from build123d import *

# Parameters (mm, degrees)
SKETCH1_R           = 9
BOSS_EXTRUDE1_DEPTH = 1.75
SKETCH2_R           = 1.67
SKETCH2_W           = 4.7
SKETCH2_H           = 4.7
CUT_EXTRUDE1_DEPTH  = 2.75


with BuildPart() as part:
    # Sketch1 → Boss-Extrude1 (new body)
    with BuildSketch(Plane.XY):
        Circle(SKETCH1_R)
    extrude(amount=BOSS_EXTRUDE1_DEPTH)

    # Sketch2 → Cut-Extrude1 (cut, through all)
    with BuildSketch(Plane.XY.offset(1.75)):
        with Locations((0, 5.25)):
            Circle(SKETCH2_R)
        Rectangle(SKETCH2_W, SKETCH2_H)
    extrude(amount=-CUT_EXTRUDE1_DEPTH, mode=Mode.SUBTRACT)


solid = part.part
The listing builds one solid part. Answer for the finished solid, in the listing's coordinates (mm). A direction names the side the tool comes from. Give positions to 0.01 mm unless a question says otherwise; leave off trailing zeros. Loops run counter-clockwise (first coordinate to the right, second up) from the corner with the lowest first, then second, coordinate; pieces in that order, holes last.
Item 1: A cutting plane is placed at A-A (x = 0). Give the vertices of the cut face in (y, z), then the cut area to 3 significant figures.
Derived:
outline: (-9, 0) - (-2.35, 0) - (-2.35, 1.75) - (-9, 1.75) - close; (2.35, 0) - (3.58, 0) - (3.58, 1.75) - (2.35, 1.75) - close; (6.92, 0) - (9, 0) - (9, 1.75) - (6.92, 1.75) - close
area: 17.4 mm2
Item 2: Each of these flat-tipped pins is pushed along its axis until it touches: pin 1 Ø5.5 at (x, y) = (0, 5.25) entering from +Z; pin 2 Ø0.9 at (x, z) = (1, 1.5) entering from -Y. Where does it stop, or does it pass through?
Derived:
pin 1: stops at z = 1.75
pin 2: stops at y = -8.98
Item 3: Determine the mould class of faces 1 (the cylindrical face through (-1.172, 8.923, 0.863)), 2 (the flat face through (-2.35, 0, 1)), 3 (the flat face through (0, -4, 1.75)) for opening direction Y: +Y half, -Y half, draft (parallel to the pull), parting line (faces both ways), or undercut.
Derived:
face 1: parting line
face 2: undercut
face 3: draft
Item 4: Find the intervals of material crossed by line 1 along Y through (x, z) = (0, 1.15); line 2 along X through (y, z) = (-0.75, 1.65); line 3 along Y through (x, z) = (2.25, 0.5), in increasing order.
Derived:
line 1: y = -9 to -2.35, 2.35 to 3.58, 6.92 to 9
line 2: x = -8.97 to -2.35, 2.35 to 8.97
line 3: y = -8.71 to -2.35, 2.35 to 8.71
Item 5: A cutting plane is placed at C-C (z = 1.35). Give the vertices of the cut face in (x, y), then the cut area to 3 significant figures.
Derived:
outline: circle Ø18 at (0, 0); hole (-2.35, -2.35) - (2.35, -2.35) - (2.35, 2.35) - (-2.35, 2.35) - close; hole circle Ø3.34 at (0, 5.25)
area: 224 mm2
Item 6: A cutting plane is placed at D-D (x = 2). Give the vertices of the cut face in (y, z), then the cut area to 3 significant figures.
Derived:
outline: (-8.77, 0) - (-2.35, 0) - (-2.35, 1.75) - (-8.77, 1.75) - close; (2.35, 0) - (8.77, 0) - (8.77, 1.75) - (2.35, 1.75) - close
area: 22.5 mm2
Item 7: A tool of negligible diameter and unlimited length cuts with its end or side. For faces 4 (the flat face through (0, -4, 0)), 5 (the flat face through (2.35, 0, 1)), from which of +Z, -Z, +X, -X, +Y, -Y can it reach the whole face along a straight path? Write none if from no direction.
Derived:
face 4: -Z, +X, -X, +Y, -Y
face 5: +Z, -Z
Item 8: A cutting plane is placed at B-B (y = 0). Give the vertices of the cut face in (x, z), then the cut area to 3 significant figures.
Derived:
outline: (-9, 0) - (-2.35, 0) - (-2.35, 1.75) - (-9, 1.75) - close; (2.35, 0) - (9, 0) - (9, 1.75) - (2.35, 1.75) - close
area: 23.3 mm2
